from build123d import *

# Parameters (mm, degrees)
EXTRUDE_590_DEPTH   = 29.1
EXTRUDE_638_DEPTH   = 9.5
FILLET_1_R          = 3
HOLE_WIZARD_M5_1_D  = 5.3
CUT_EXTRUDE_1_DEPTH = 5
CUT_EXTRUDE_2_DEPTH = 0.5


with BuildPart() as part:
    # 草图1 → Extrude 590 (new body)
    with BuildSketch(Plane(origin=(0, 0, 0), x_dir=(1, 0, 0), z_dir=(0, 1, 0))):
        with BuildLine():
            Line((4.608867317, -165), (-4.608867317, -165))
            Line((-4.608867317, -165), (-5.444719551, -194.923972433))
            ThreePointArc((-5.444719551, -194.923972433), (0, -195), (5.444719551, -194.923972433))
            Line((5.444719551, -194.923972433), (4.608867317, -165))
        make_face()
    extrude(amount=EXTRUDE_590_DEPTH)

    # 草图1<3> → Extrude 638 (add)
    with BuildSketch(Plane(origin=(0, 0, 0), x_dir=(1, 0, 0), z_dir=(0, 1, 0))):
        with BuildLine():
            ThreePointArc((5.444719551, -194.923972433), (0, -195), (-5.444719551, -194.923972433))
            Line((-5.444719551, -194.923972433), (-5.584327745, -199.922023008))
            ThreePointArc((-5.584327745, -199.922023008), (0, -200), (5.584327745, -199.922023008))
            Line((5.584327745, -199.922023008), (5.444719551, -194.923972433))
        make_face()
    extrude(amount=EXTRUDE_638_DEPTH)

    # 圆角1
    fillet_1_edges = [part.edges().sort_by_distance(p)[0] for p in [
        (4.608867317, 14.55, 165),
        (0, 0, 165),
        (-4.608867317, 14.55, 165),
    ]]
    fillet(fillet_1_edges, radius=FILLET_1_R)

    # M5 间隙孔1 (through all)
    with Locations(Plane(origin=(0, 29.1, 0), x_dir=(1, 0, 0), z_dir=(0, 1, 0))):
        with Locations((0, -187), (0, -175)):
            Hole(HOLE_WIZARD_M5_1_D / 2)

    # 草图6 → 切除-拉伸1 (cut)
    with BuildSketch(Plane.XZ):
        Polygon((0, 179.618802154), (-4, 177.309401077), (-4, 172.690598923), (0, 170.381197846), (4, 172.690598923), (4, 177.309401077), align=None)
        Polygon((0, 191.618802154), (-4, 189.309401077), (-4, 184.690598923), (0, 182.381197846), (4, 184.690598923), (4, 189.309401077), align=None)
    extrude(amount=-CUT_EXTRUDE_1_DEPTH, mode=Mode.SUBTRACT)

    # 草图7 → 切除-拉伸2 (cut)
    with BuildSketch(Plane(origin=(0, 0, 0), x_dir=(-0.027921638723569116, 0, -0.9996101150403545), z_dir=(0.9996101150403545, 0, -0.027921638723569116))):
        Polygon((-172.103223024, 27.6), (-171.456087608, 27.6), (-171.456087608, 24.1), (-171.770190172, 24.1), (-171.770190172, 27.241025641), (-172.30865171, 27.241025641), align=None)
    extrude(amount=-CUT_EXTRUDE_2_DEPTH, mode=Mode.SUBTRACT)


solid = part.part
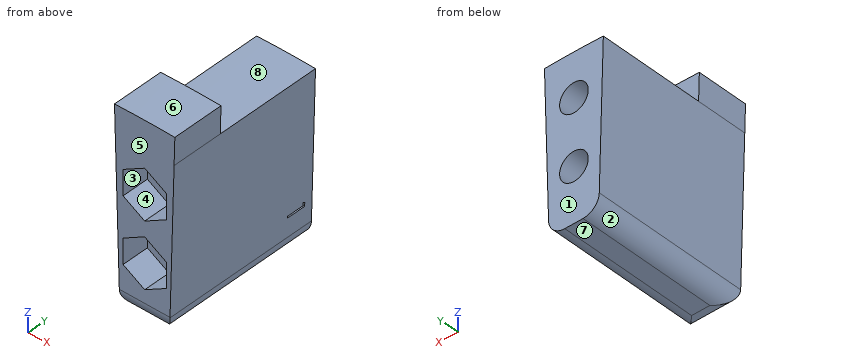
Input: part model. Units: mm. Frame: model coordinates. Face numbers are marked on the shaded views. A direction names the side the tool comes from. Round coordinates to 2 decimals unless told otherwise and drop trailing zeros. Order: outer loops, then holes, each group sorted by start corner. A loop starts at its lowest first (then second) coordinate and runs counter-clockwise, first axis right, second up. Notation, with made-up numbers: (71.5, 37) - (114.5, 37) arc R7 cw to (114.5, 45) - close; hole circle Ø5 at (71.5, 54). An arc over 180 degrees is marked (long way). Answer as a JSON object with one key per item and string values. Group by question number.
(1) Cut plane D-D (z = 187). Return loops of the section in (x, y).
(2) Pin query (flat end, axial travel): P1, Ø3.5, axis at y = 3.5, z = 174, coming from the -X side; P2, Ø1.4, axis at y = 1.5, z = 188, coming from the +X side; P3, Ø3, axis at y = 22, z = 194, coming from the +X side; P4, Ø4, axis at x = -1, z = 175.5, coming from the +Y side. Return the tip coordinate at first contact, or that it passes through.
(3) Material intervals for probe 1 along Z at (x, y) = (0, 13.5); probe 2 along Z at (x, y) = (-1.5, 2); probe 3 along Y at (x, z) = (0.25, 197), sorted ascending. Write a range as from..to.
(4) Cut plane C-C (x = -2.25). Return loops of the section in (y, z).
(5) Cut plane A-A (y = 23). Return loops of the section in (x, z), then the cut area to 3 significant figures.
(6) Reachability of the marked faces 4, 5, 6, 7 and 8 from +Z, -Z, +X, -X, +Y, -Y: full face, straight path, thin tool, end or side. Return the list, or none.
(7) Draft query along X for the marked faces 1, 2 and 3. Return one class per face: released by +X, released by -X, zero draft, split by the parting line, or undercut.
(8) Cut plane B-B (z = 175.5). Return loops of the section in (x, y), then the cut area to 3 significant figures.
Here are the results:
{
 "1": {"outline": "(-5.22, 0) - (-4, 0) - (-4, 5) - (-2.65, 5) - (-2.65, 29.1) - (-5.22, 29.1) - close; (2.65, 5) - (4, 5) - (4, 0) - (5.22, 0) - (5.22, 29.1) - (2.65, 29.1) - close"},
 "2": {"P1": "stops at x = -4.91", "P2": "stops at x = 5.27", "P3": "stops at x = 5.44", "P4": "stops at y = 29.1"},
 "3": {"probe 1": "z = 165..172.35, 177.65..184.35, 189.65..195", "probe 2": "z = 165.17..171.25, 178.75..183.25, 190.75..199.99", "probe 3": "y = 0..9.5"},
 "4": {"outline": "(0, 168) arc R3 ccw to (2.44, 165.05) - (29.1, 165.05) - (29.1, 173.6) - (5, 173.6) - (5, 171.68) - (0, 171.68) - close; (0, 178.32) - (5, 178.32) - (5, 176.4) - (29.1, 176.4) - (29.1, 185.6) - (5, 185.6) - (5, 183.68) - (0, 183.68) - close; (0, 190.32) - (5, 190.32) - (5, 188.4) - (29.1, 188.4) - (29.1, 194.99) - (9.5, 194.99) - (9.5, 199.99) - (0, 199.99) - close"},
 "5": {"outline": "(-5.44, 194.92) - (-4.69, 167.92) arc R3 ccw to (-1.69, 165) - (1.69, 165) arc R3 ccw to (4.69, 167.92) - (5.44, 194.92) arc R195 ccw to start; hole circle Ø5.3 at (0, 175); hole circle Ø5.3 at (0, 187)", "area": "254 mm^2"},
 "6": {"face 4": "-Y", "face 5": "+Z, -Z, +X, -X, -Y", "face 6": "+Z, +Y, -Y", "face 7": "-Z, +X, -X, +Y, -Y", "face 8": "+Z, +Y"},
 "7": {"face 1": "zero draft", "face 2": "released by -X", "face 3": "undercut"},
 "8": {"outline": "(-4.9, 0) - (-4, 0) - (-4, 5) - (-2.6, 5) - (-2.6, 29.1) - (-4.9, 29.1) - close; (2.6, 5) - (4, 5) - (4, 0) - (4.9, 0) - (4.9, 29.1) - (2.6, 29.1) - close", "area": "120 mm^2"}
}
